Verification items for the finished model (mm, model axes). Round coordinates to 2 decimals unless told otherwise and drop trailing zeros. Write each loop counter-clockwise with the first axis right and the second up, starting at its lowest first coordinate (ties: lowest second). Pieces come first, ordered by that corner, then holes. Notation, with made-up numbers: M 43.25,66 L 51.25,66 A30 ccw 51.25,92 Z; hole C 74,26 d11. An arc over 180 degrees is marked long. One line per question, with ' | ' between items.
from build123d import *

# Parameters (mm, degrees)
SKETCH1_W           = 231.775
SKETCH1_H           = 6.350433672
SKETCH1_W_2         = 6.35
SKETCH1_H_2         = 76.2
SKETCH1_H_3         = 12.7
SKETCH1_W_3         = 3.175
BOSS_EXTRUDE1_DEPTH = 6.35
CUT_EXTRUDE1_DEPTH  = 341.219392139
FILLET1_R           = 0.635
SKETCH3_R           = 0.889
CUT_EXTRUDE2_DEPTH  = 341.219392139


with BuildPart() as part:
    # Sketch1 → Boss-Extrude1 (new body)
    with BuildSketch(Plane(origin=(0, 0, 0), x_dir=(1, 0, 0), z_dir=(0, 1, 0))):
        with Locations((184.959182845, 155.570446755)):
            Rectangle(SKETCH1_W, SKETCH1_H)
        with BuildLine():
            Line((69.071682845, 152.395229919), (69.071682845, 158.745663591))
            ThreePointArc((69.071682845, 158.745663591), (20.184176976, 138.015461144), (0, 88.9))
            Line((0, 88.9), (6.35, 88.9))
            ThreePointArc((6.35, 88.9), (24.674380805, 133.525255521), (69.071682845, 152.395229919))
        make_face()
        with Locations((3.175, 50.8)):
            Rectangle(SKETCH1_W_2, SKETCH1_H_2)
        with Locations((3.175, 6.35)):
            Rectangle(SKETCH1_W_2, SKETCH1_H_3)
        with Locations((-1.5875, 6.35)):
            Rectangle(SKETCH1_W_3, SKETCH1_H_3)
        with Locations((7.9375, 6.35)):
            Rectangle(SKETCH1_W_3, SKETCH1_H_3)
    extrude(amount=BOSS_EXTRUDE1_DEPTH)

    # Sketch2 → Cut-Extrude1 (cut, through all)
    with BuildSketch(Plane(origin=(0, 6.35, 0), x_dir=(1, 0, 0), z_dir=(0, 1, 0))):
        Polygon((3.175, 0), (-3.175, 12.7), (-3.175, 0), align=None)
        Polygon((9.525, 12.7), (3.175, 0), (9.525, 0), align=None)
    extrude(amount=-CUT_EXTRUDE1_DEPTH, mode=Mode.SUBTRACT)

    # Fillet1
    fillet1_edges = [part.edges().sort_by_distance(p)[0] for p in [
        (0, 3.175, -12.7),
        (300.846682845, 3.175, -158.745663591),
        (300.846682845, 3.175, -152.395229919),
        (6.35, 3.175, -12.7),
        (-3.175, 3.175, -12.7),
        (9.525, 3.175, -12.7),
        (3.175, 3.175, 0),
    ]]
    fillet(fillet1_edges, radius=FILLET1_R)

    # Sketch3 → Cut-Extrude2 (cut, through all)
    with BuildSketch(Plane(origin=(0, 6.35, 0), x_dir=(1, 0, 0), z_dir=(0, 1, 0))):
        with Locations(Location((3.175, 26.184903166, 0), (0, 0, 270))):
            Circle(SKETCH3_R)
        with Locations(Location((3.175, 89.684903166, 0), (0, 0, 270))):
            Circle(SKETCH3_R)
        with Locations(Location((66.802, 155.570446755, 0), (0, 0, 270))):
            Circle(SKETCH3_R)
        with Locations(Location((270.002, 155.570446755, 0), (0, 0, 270))):
            Circle(SKETCH3_R)
    extrude(amount=-CUT_EXTRUDE2_DEPTH, mode=Mode.SUBTRACT)


solid = part.part
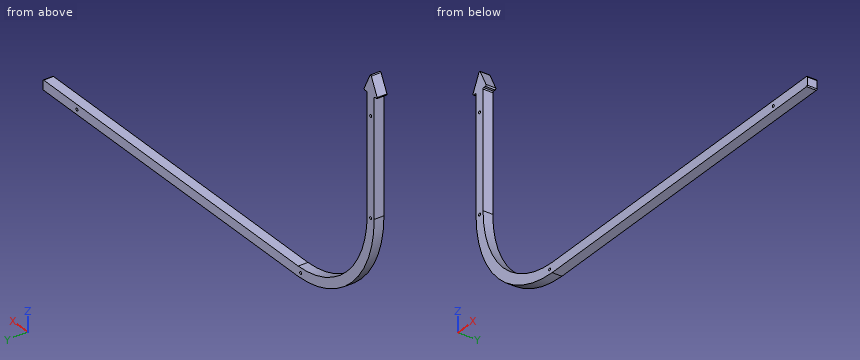
1. Section check B-B, the plane z = -76. Record the cut outline in (x, y), then the cut area to 3 significant figures.
Results:
outline: M 0,0 L 6.35,0 L 6.35,6.35 L 0,6.35 Z | area: 40.3 mm2
2. Go/stop test with flat-tipped pins: P1, Ø1.9, axis at y = 4, z = -62.5, coming from the +X side; P2, Ø0.5, axis at x = 8, y = 4, coming from the -Z side; P3, Ø1.9, axis at x = 223, y = 2.5, coming from the +Z side. Record where each tip stops, or that it passes through.
Results:
P1: stops at x = 6.35 | P2: stops at z = -121.83 | P3: stops at z = -152.4
3. Thickness scan on line 1 (Z direction, x = 162, y = 5.5); line 2 (X direction, y = 2.5, z = -70.5); line 3 (X direction, y = 2.5, z = -11.5) (3 decimals). Record the ranges inside material, lowest first.
Results:
line 1: z = -158.75 to -152.4 | line 2: x = 0 to 6.35 | line 3: x = -2.575 to 8.925
4. Section check C-C, the plane x = 230. Record the cut outline in (y, z), then the cut area to 3 significant figures.
Results:
outline: M 0,-158.75 L 6.35,-158.75 L 6.35,-152.4 L 0,-152.4 Z | area: 40.3 mm2
5. Section check A-A, the plane y = 3. Count the separate pieces of the cut face and the enclosed holes in it, then the cut area to 3 significant figures.
Results:
separate pieces: 1 | enclosed holes: 4 | area: 2,690 mm2
